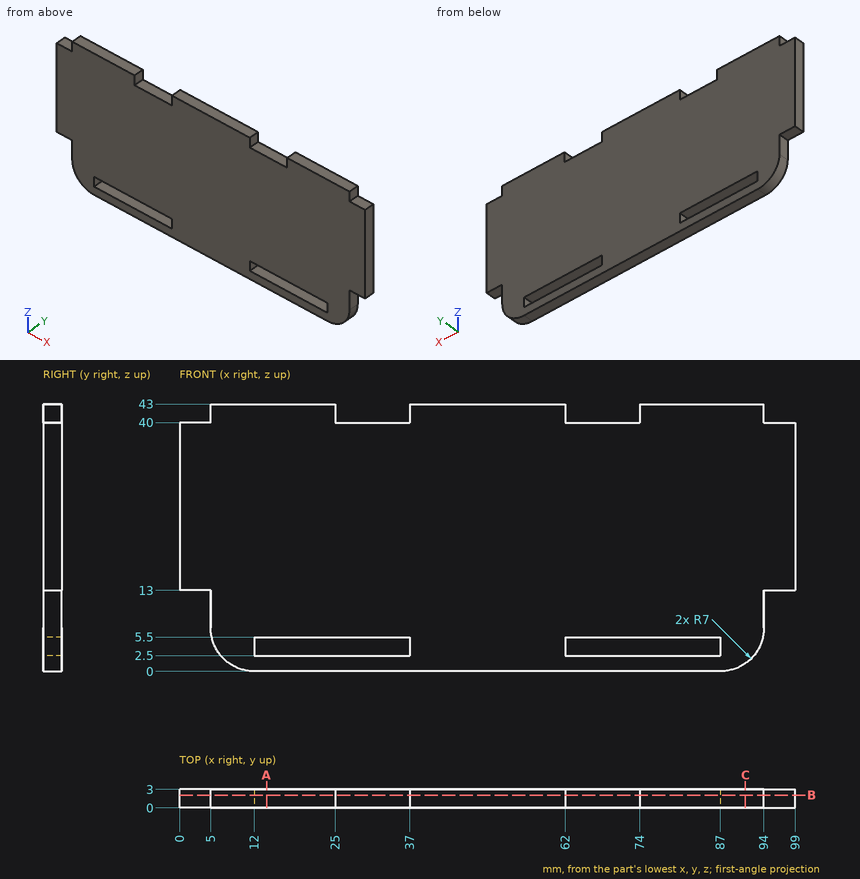
Geometry check sheet. Reference: drawing and pictorial views, mm from the part's lowest x, y, z. Round coordinates to 2 decimals unless told otherwise and drop trailing zeros. Loops run counter-clockwise (first coordinate to the right, second up) from the corner with the lowest first, then second, coordinate; pieces in that order, holes last. Notation, with made-up numbers: M -23.75,-30 L 6.25,-30 A16 cw 6.25,-14 Z; hole C 40.25,9.5 d1. An arc over 180 degrees is marked long. One line per item, written item: value.
(1) Thickness scan on line 1 (X direction, y = 1.6, z = 4); line 2 (Z direction, x = 14, y = 0.2); line 3 (Z direction, x = 65.5, y = 1.1). Record the ranges inside material, lowest first.
Computed values:
line 1: x = 5.68 to 12, 37 to 62, 87 to 93.32
line 2: z = 0 to 2.5, 5.5 to 43
line 3: z = 0 to 2.5, 5.5 to 40
(2) Depth check by flat-ended pin: pin 1 Ø1.5 at (y, z) = (1.5, 4) entering from -X; pin 2 Ø1.5 at (y, z) = (1, 42) entering from -X; pin 3 Ø1.5 at (x, y) = (97, 1.5) entering from -Z; pin 4 Ø8 at (x, z) = (51, 37.5) entering from -Y. Enter the tip coordinate at first touch or a pass-through.
Computed values:
pin 1: stops at x = 5.37
pin 2: stops at x = 5
pin 3: stops at z = 13
pin 4: stops at y = 0
(3) Sectioned sample at A-A, the plane x = 14. Record the cut outline in (y, z).
Computed values:
outline: M 0,0 L 3,0 L 3,2.5 L 0,2.5 Z; M 0,5.5 L 3,5.5 L 3,43 L 0,43 Z
(4) Sectioned sample at C-C, the plane x = 91. Record the cut outline in (y, z), then the cut area to 3 significant figures.
Computed values:
outline: M 0,1.26 L 3,1.26 L 3,43 L 0,43 Z
area: 125 mm^2
(5) Sectioned sample at B-B, the plane y = 2.05. Count the separate pieces of the cut face and the enclosed holes in it, then the cut area to 3 significant figures.
Computed values:
separate pieces: 1
enclosed holes: 2
area: 3,850 mm^2
